Input: part model. Units: mm. Frame: model coordinates. A direction names the side the tool comes from. Give positions to 0.01 mm unless a question says otherwise; leave off trailing zeros. Write each loop counter-clockwise with the first axis right and the second up, starting at its lowest first coordinate (ties: lowest second). Pieces come first, ordered by that corner, then holes. Notation, with made-up numbers: (36, 54) -> (86, 54) arc R21 cw to (86, 85) -> close; hole circle Ø6 at (11.5, 68). An arc over 180 degrees is marked (long way). Return JSON: item names as keys, results as strings. Group by question number.
Item 1: Line query: line 1 (X direction, y = 55, z = 33); line 2 (Z direction, x = 42, y = 36.5). Output: solid intervals per line, ascending. Write a range as [from, to].
Item 2: Section C-C, the plane x = -10. Return loops of the section in (y, z).
Item 3: Section A-A, the plane z = 52.5. Return loops of the section in (x, y).
Item 4: Pin query (flat end, axial travel): P1, Ø10, axis at x = -7, y = 24.5, coming from the +Z side. Return the tip coordinate at first contact, or that it passes through.
Item 5: Mould query, pull axis X, two halves, no side actions, for faces 3 (the face through (-1, 1, 1.5)), 4 (the face through (-1, 1, 0)), 5 (the face through (-50, -1, 39)), 6 (the face through (-48.5, -1, 40)). Classes: released by +X, released by -X, zero draft, split by the parting line, or undercut.
Item 6: Section B-B, the plane y = -15.5. Return loops of the section in (x, z), then the cut area to 4 significant figures.
Item 7: Set-up query: faces 1 (the face through (0, -100, 1)), 2 (the face through (48.5, -1, 40)). Return all of +Z, -Z, +X, -X, +Y, -Y with unobstructed straight access to the full face (end or side cutting, diameter ignored); none if empty.
from build123d import *

# Parameters (mm, degrees)
SKETCH1_W           = 100
SKETCH1_H           = 200
BOSS_EXTRUDE1_DEPTH = 80
SHELL1_T            = -1.5


with BuildPart() as part:
    # Sketch1 → Boss-Extrude1 (new body)
    with BuildSketch(Plane.XY):
        Rectangle(SKETCH1_W, SKETCH1_H)
    extrude(amount=BOSS_EXTRUDE1_DEPTH)

    # Shell1
    shell1_openings = [part.faces().sort_by_distance(p)[0] for p in [
        (0, 0, 80),
        (0, 100, 40),
        (0, -100, 40),
    ]]
    offset(amount=SHELL1_T, openings=shell1_openings, kind=Kind.INTERSECTION)


solid = part.part
Answer below:
{
 "1": {"line 1": "x = [-50, -48.5], [48.5, 50]", "line 2": "z = [0, 1.5]"},
 "2": {"outline": "(-100, 0) -> (100, 0) -> (100, 1.5) -> (-100, 1.5) -> close"},
 "3": {"outline": "(-50, -100) -> (-48.5, -100) -> (-48.5, 100) -> (-50, 100) -> close; (48.5, -100) -> (50, -100) -> (50, 100) -> (48.5, 100) -> close"},
 "4": {"P1": "stops at z = 1.5"},
 "5": {"face 3": "undercut", "face 4": "zero draft", "face 5": "released by -X", "face 6": "undercut"},
 "6": {"outline": "(-50, 0) -> (50, 0) -> (50, 80) -> (48.5, 80) -> (48.5, 1.5) -> (-48.5, 1.5) -> (-48.5, 80) -> (-50, 80) -> close", "area": "385.5 mm2"},
 "7": {"face 1": "+Z, -Z, +X, -X, -Y", "face 2": "+Z, +Y, -Y"}
}
